from build123d import *

# Parameters (mm, degrees)
CROQUIS1_W                         = 35
CROQUIS1_H                         = 36
BRIDA_BASE1_DEPTH                  = 1.2
BRIDA_DE_ARISTA1_STRIP_W           = 6.2732
BRIDA_DE_ARISTA1_STRIP_H           = 1.2
BRIDA_DE_ARISTA1_STRIP_CUT_DEPTH   = 36
BRIDA_DE_ARISTA1_STRIP_2_W         = 6.2732
BRIDA_DE_ARISTA1_STRIP_2_H         = 1.2
BRIDA_DE_ARISTA1_STRIP_CUT_2_DEPTH = 36
BRIDA_DE_ARISTA1_DEPTH             = 36
BRIDA_DE_ARISTA1_BEND_DEPTH        = 36
CROQUIS14_W                        = 36
CROQUIS14_H                        = 7
CORTAR_EXTRUIR3_DEPTH              = 1.2
CROQUIS12_R                        = 2
CORTAR_EXTRUIR1_DEPTH              = 1.2
CROQUIS13_R                        = 4
CORTAR_EXTRUIR2_DEPTH              = 1.2
REDONDEO1_R                        = 5


# Sheet-metal steps are written as plain solids
with BuildPart() as part:
    # Croquis1 → Brida base1 (new body)
    with BuildSketch(Plane(origin=(0, 0, 0), x_dir=(1, 0, 0), z_dir=(0, 1, 0))):
        Rectangle(CROQUIS1_W, CROQUIS1_H)
    extrude(amount=-BRIDA_BASE1_DEPTH)

    # Brida de arista1 strip (across the edge) → Brida de arista1 strip cut (cut)
    with BuildSketch(Plane(origin=(17.5, 0, 18), x_dir=(-1, 0, 0), z_dir=(0, 0, -1))):
        with Locations((-1.2, -0.6)):
            Rectangle(BRIDA_DE_ARISTA1_STRIP_W, BRIDA_DE_ARISTA1_STRIP_H)
    extrude(amount=BRIDA_DE_ARISTA1_STRIP_CUT_DEPTH, mode=Mode.SUBTRACT)

    # Brida de arista1 strip 2 (across the edge) → Brida de arista1 strip cut 2 (cut)
    with BuildSketch(Plane(origin=(-17.5, 0, -18), x_dir=(1, 0, 0), z_dir=(0, 0, 1))):
        with Locations((-1.2, -0.6)):
            Rectangle(BRIDA_DE_ARISTA1_STRIP_2_W, BRIDA_DE_ARISTA1_STRIP_2_H)
    extrude(amount=BRIDA_DE_ARISTA1_STRIP_CUT_2_DEPTH, mode=Mode.SUBTRACT)

    # Brida de arista1 section (across the edge) → Brida de arista1 (add)
    with BuildSketch(Plane(origin=(17.5, 0, 18), x_dir=(-1, 0, 0), z_dir=(0, 0, -1))):
        with BuildLine():
            Line((0, 0.7366), (0, 29.8))
            Line((0, 29.8), (1.2, 29.8))
            Line((1.2, 29.8), (1.2, 0.7366))
            ThreePointArc((1.2, 0.7366), (1.415745145, 0.215745145), (1.9366, 0))
            Line((1.9366, 0), (1.9366, -1.2))
            ThreePointArc((1.9366, -1.2), (0.567217008, -0.632782992), (0, 0.7366))
        make_face()
    extrude(amount=BRIDA_DE_ARISTA1_DEPTH)

    # Brida de arista1 section 2 (across the edge) → Brida de arista1 bend (add)
    with BuildSketch(Plane(origin=(-17.5, 0, -18), x_dir=(1, 0, 0), z_dir=(0, 0, 1))):
        with BuildLine():
            Line((0, 0.7366), (0, 29.8))
            Line((0, 29.8), (1.2, 29.8))
            Line((1.2, 29.8), (1.2, 0.7366))
            ThreePointArc((1.2, 0.7366), (1.415745145, 0.215745145), (1.9366, 0))
            Line((1.9366, 0), (1.9366, -1.2))
            ThreePointArc((1.9366, -1.2), (0.567217008, -0.632782992), (0, 0.7366))
        make_face()
    extrude(amount=BRIDA_DE_ARISTA1_BEND_DEPTH)

    # Croquis14 → Cortar-Extruir3 (cut)
    with BuildSketch(Plane(origin=(17.5, 0, 0), x_dir=(0, 0, -1), z_dir=(1, 0, 0))):
        with Locations((0, 26.3)):
            Rectangle(CROQUIS14_W, CROQUIS14_H)
    extrude(amount=-CORTAR_EXTRUIR3_DEPTH, mode=Mode.SUBTRACT)

    # Croquis12 → Cortar-Extruir1 (cut)
    with BuildSketch(Plane(origin=(17.5, 0, 0), x_dir=(0, 0, -1), z_dir=(1, 0, 0))):
        with Locations(Location((-12.5, 18.05, 0), (0, 0, 90))):
            Circle(CROQUIS12_R)
        with Locations(Location((12.5, 18.05, 0), (0, 0, 90))):
            Circle(CROQUIS12_R)
        with Locations(Location((0, 5.55, 0), (0, 0, 90))):
            Circle(CROQUIS12_R)
    extrude(amount=-CORTAR_EXTRUIR1_DEPTH, mode=Mode.SUBTRACT)

    # Croquis13 → Cortar-Extruir2 (cut)
    with BuildSketch(Plane(origin=(-16.3, 0, 0), x_dir=(0, 0, -1), z_dir=(1, 0, 0))):
        with Locations(Location((0, 15.2683, 0), (0, 0, 90))):
            Circle(CROQUIS13_R)
    extrude(amount=-CORTAR_EXTRUIR2_DEPTH, mode=Mode.SUBTRACT)

    # Redondeo1
    redondeo1_edges = [part.edges().sort_by_distance(p)[0] for p in [
        (-16.9, 29.8, -18),
        (-16.9, 29.8, 18),
        (16.9, 22.8, 18),
        (16.9, 22.8, -18),
    ]]
    fillet(redondeo1_edges, radius=REDONDEO1_R)


solid = part.part
Part model, mm, in its own coordinate system. A direction names the side the tool comes from. Coordinates: 2 decimals unless noted, no trailing zeros. Order: outer loops, then holes, each group sorted by start corner. A loop starts at its lowest first (then second) coordinate and runs counter-clockwise, first axis right, second up. Notation, with made-up numbers: (11, -11) - (65, -11) arc R19 cw to (65, 17) - close; hole circle Ø11 at (56.5, 51). An arc over 180 degrees is marked (long way). Use CSV: the item, a comma, the result in double quotes.
Item 1: 3-axis set-ups, long thin cutter, end or side, ignore diameter. For faces 1 (the face through (16.89, 21.3, 16.57)), 2 (the face through (17, 22.8, 0)), 3 (the face through (-16.3, 15.5, -4.3)), 4 (the face through (16.908, 16.052, 12.588)), 5 (the face through (16.89, 21.3, -16.57)): which of +Z, -Z, +X, -X, +Y, -Y reach the whole face in a straight line?
Solved:
face 1,"+Z, +X, +Y"
face 2,"+Z, -Z, +X, +Y"
face 3,"+Z, -Z, +Y"
face 4,"+X"
face 5,"-Z, +X, +Y"
Item 2: Probe probe 1 along Z at (x, y) = (17.2, 18.05); probe 2 along X at (y, z) = (10, 13); probe 3 along Z at (x, y) = (17.2, 5.55). List the from-to ranges inside material, lowest first.
Solved:
probe 1,"z = -17.99 to -14.5, -10.5 to 10.5, 14.5 to 17.99"
probe 2,"x = -17.5 to -16.3, 16.3 to 17.5"
probe 3,"z = -18 to -2, 2 to 18"
Item 3: Saw through at A-A on y = 5.55. Give the cut face in (x, z), and give its area (3 significant figures).
Solved:
outline,"(-17.5, -18) - (-16.3, -18) - (-16.3, 18) - (-17.5, 18) - close; (16.3, -18) - (17.5, -18) - (17.5, -2) - (16.3, -2) - close; (16.3, 2) - (17.5, 2) - (17.5, 18) - (16.3, 18) - close"
area,"81.6 mm²"
Item 4: Saw through at D-D on z = -10. Give the cut face in (x, y), and give its area (3 significant figures).
Solved:
outline,"(-17.5, 0.74) arc R1.94 ccw to (-15.56, -1.2) - (15.56, -1.2) arc R1.94 ccw to (17.5, 0.74) - (17.5, 22.8) - (16.3, 22.8) - (16.3, 0.74) arc R0.74 cw to (15.56, 0) - (-15.56, 0) arc R0.74 cw to (-16.3, 0.74) - (-16.3, 29.8) - (-17.5, 29.8) - close"
area,"104 mm²"
Item 5: Saw through at B-B on z = 0. Give the cut face in (x, y).
Solved:
outline,"(-17.5, 0.74) arc R1.94 ccw to (-15.56, -1.2) - (15.56, -1.2) arc R1.94 ccw to (17.5, 0.74) - (17.5, 3.55) - (16.3, 3.55) - (16.3, 0.74) arc R0.74 cw to (15.56, 0) - (-15.56, 0) arc R0.74 cw to (-16.3, 0.74) - (-16.3, 11.27) - (-17.5, 11.27) - close; (-17.5, 19.27) - (-16.3, 19.27) - (-16.3, 29.8) - (-17.5, 29.8) - close; (16.3, 7.55) - (17.5, 7.55) - (17.5, 22.8) - (16.3, 22.8) - close"
Item 6: Mould opens along Z. For faces 6 (the face through (-1, -1, -18)), 7 (the face through (0, 0, 0)), 8 (the face through (16.908, 7.397, -0.766)) say: +Z half, -Z half, draft (parallel to the pull), parting line (faces both ways), or undercut.
Solved:
face 6,"-Z half"
face 7,"draft"
face 8,"undercut"
Item 7: Drop flat-ended pins along their axis: P1, Ø4.5, axis at y = 18.05, z = -12.5, coming from the +X side; P2, Ø15.5, axis at x = 4.5, z = 5, coming from the +Y side; P3, Ø2, axis at y = 18.5, z = -13, coming from the +X side; P4, Ø5, axis at y = 15.27, z = 0, coming from the -X side. Give the stop position or say it passes through.
Solved:
P1,"stops at x = 17.5"
P2,"stops at y = 0"
P3,"stops at x = -16.3"
P4,"stops at x = 16.3"
Item 8: Saw through at C-C on z = 12.5. Give the cut face in (x, y).
Solved:
outline,"(-17.5, 0.74) arc R1.94 ccw to (-15.56, -1.2) - (15.56, -1.2) arc R1.94 ccw to (17.5, 0.74) - (17.5, 16.05) - (16.3, 16.05) - (16.3, 0.74) arc R0.74 cw to (15.56, 0) - (-15.56, 0) arc R0.74 cw to (-16.3, 0.74) - (-16.3, 29.8) - (-17.5, 29.8) - close; (16.3, 20.05) - (17.5, 20.05) - (17.5, 22.8) - (16.3, 22.8) - close"
